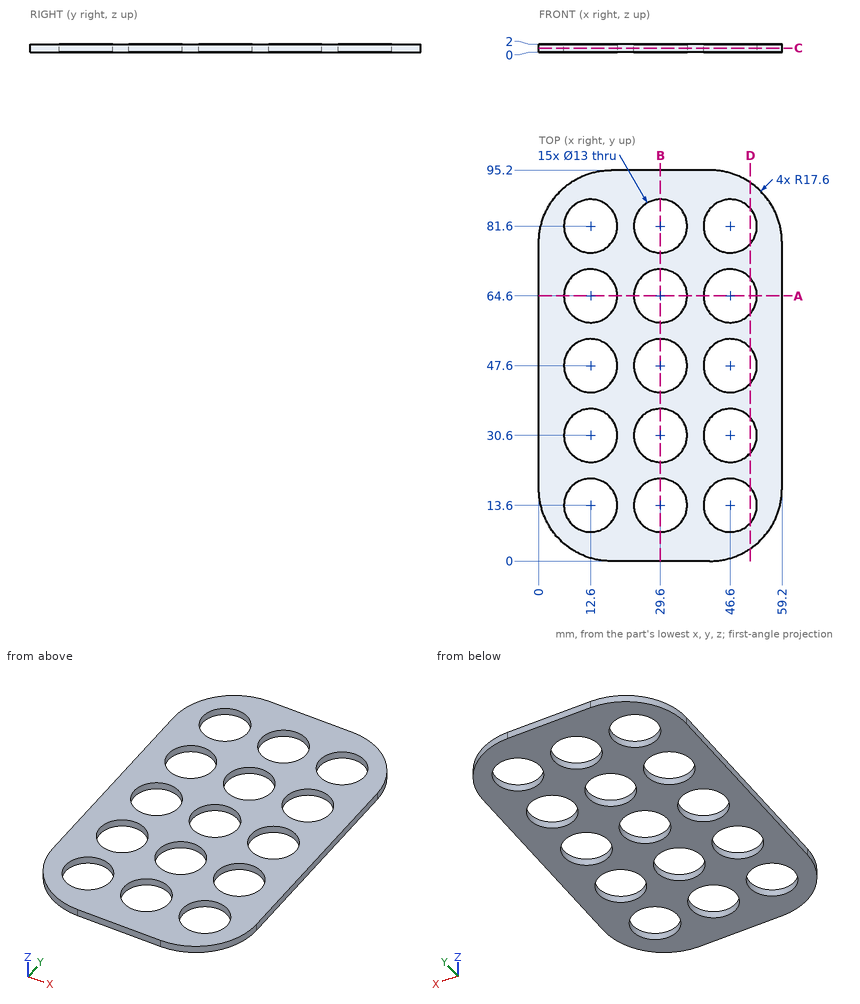
Verification items for this drawing (mm, ordinates from the low corner). Coordinates: 2 decimals unless noted, no trailing zeros. Write each loop counter-clockwise with the first axis right and the second up, starting at its lowest first coordinate (ties: lowest second). Pieces come first, ordered by that corner, then holes. Notation, with made-up numbers: M 14,23 L 27,23 A16 ccw 27,32 Z; hole C -1.5,17 d3. An arc over 180 degrees is marked long. Use one line per item in the form item = value. Start each with the question number.
1) Section check C-C on z = 1. State how many separate pieces and enclosed holes the cut face has, and give its area (3 significant figures).
2) Thickness scan on probe 1 along Y at (x, z) = (29.6, 1.5); probe 2 along Y at (x, z) = (7, 1.55); probe 3 along X at (y, z) = (63, 1.6). Record the ranges inside material, lowest first. Write a range as from..to.
3) Section check D-D on x = 51.5. Enter the section's corners in (y, z).
4) Section check B-B on x = 29.6. Enter the section's corners in (y, z), and give its area (3 significant figures).
5) Section check A-A on y = 64.6. Enter the section's corners in (x, z).
6) Go/stop test with a flat-tipped pin: pin 1 Ø11.5 at (x, y) = (46.6, 81.6) entering from -Z. Record where the tip stops, or that it passes through.
Responses:
q1.separate_pieces = 1
q1.enclosed_holes = 15
q1.area = 3,380 mm2
q2.probe_1 = 0..7.1, 20.1..24.1, 37.1..41.1, 54.1..58.1, 71.1..75.1, 88.1..95.2
q2.probe_2 = 3.55..10.3, 16.9..27.3, 33.9..44.3, 50.9..61.3, 67.9..78.3, 84.9..91.65
q2.probe_3 = 0..6.3, 18.9..23.3, 35.9..40.3, 52.9..59.2
q3.outline = M 3.05,0 L 9.33,0 L 9.33,2 L 3.05,2 Z; M 17.87,0 L 26.33,0 L 26.33,2 L 17.87,2 Z; M 34.87,0 L 43.33,0 L 43.33,2 L 34.87,2 Z; M 51.87,0 L 60.33,0 L 60.33,2 L 51.87,2 Z; M 68.87,0 L 77.33,0 L 77.33,2 L 68.87,2 Z; M 85.87,0 L 92.15,0 L 92.15,2 L 85.87,2 Z
q4.outline = M 0,0 L 7.1,0 L 7.1,2 L 0,2 Z; M 20.1,0 L 24.1,0 L 24.1,2 L 20.1,2 Z; M 37.1,0 L 41.1,0 L 41.1,2 L 37.1,2 Z; M 54.1,0 L 58.1,0 L 58.1,2 L 54.1,2 Z; M 71.1,0 L 75.1,0 L 75.1,2 L 71.1,2 Z; M 88.1,0 L 95.2,0 L 95.2,2 L 88.1,2 Z
q4.area = 60.4 mm2
q5.outline = M 0,0 L 6.1,0 L 6.1,2 L 0,2 Z; M 19.1,0 L 23.1,0 L 23.1,2 L 19.1,2 Z; M 36.1,0 L 40.1,0 L 40.1,2 L 36.1,2 Z; M 53.1,0 L 59.2,0 L 59.2,2 L 53.1,2 Z
q6.pin_1 = through
